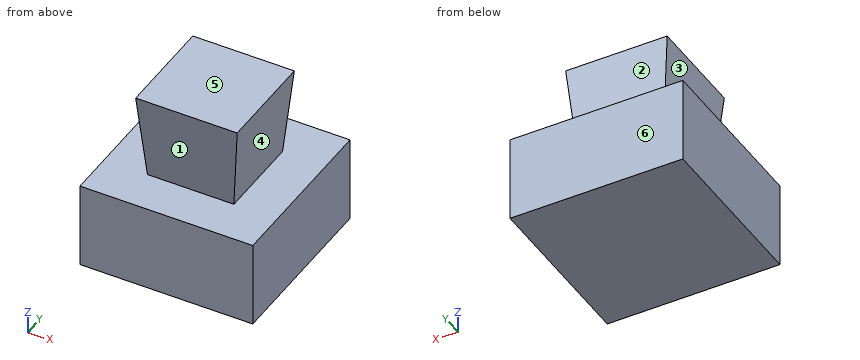
from build123d import *

# Parameters (mm, degrees)
SKETCH_1_W         = 20
SKETCH_1_H         = 20
BASEBOX_DEPTH      = 10
SKETCH_2_W         = 10
SKETCH_2_H         = 10
DRAFTOUTWARD_DEPTH = 10
DRAFTOUTWARD_DRAFT = -5


with BuildPart() as part:
    # 草图1 → BaseBox (new body)
    with BuildSketch(Plane.XY):
        with Locations((10, 10)):
            Rectangle(SKETCH_1_W, SKETCH_1_H)
    extrude(amount=BASEBOX_DEPTH)


with BuildPart() as draftoutward_tool:
    # 草图2 → DraftOutward (with draft: the straight prism first)
    with BuildSketch(Plane.XY.offset(10)):
        with Locations((10, 10)):
            Rectangle(SKETCH_2_W, SKETCH_2_H)
    extrude(amount=DRAFTOUTWARD_DEPTH)
    # DraftOutward: the draft: its side faces are tilted about the plane it starts from
    draftoutward_sides = [draftoutward_tool.faces().sort_by_distance(p)[0] for p in [
        (10, 5, 15),
        (15, 10, 15),
        (10, 15, 15),
        (5, 10, 15),
    ]]
    draft(draftoutward_sides, Plane.XY.offset(10), DRAFTOUTWARD_DRAFT)


with BuildPart() as part_1:
    add(part.part)

    # DraftOutward: add draftoutward_tool
    add(draftoutward_tool.part)


solid = part_1.part
Input: part model. Units: mm. Frame: model coordinates. Face numbers are marked on the shaded views. A direction names the side the tool comes from. Coordinates: 2 decimals unless noted, no trailing zeros. Loops run counter-clockwise (first coordinate to the right, second up) from the corner with the lowest first, then second, coordinate; pieces in that order, holes last. Notation, with made-up numbers: (0, -4.5) -> (45, -4.5) arc R30 cw to (45, 28.5) -> close; hole circle Ø6 at (14.25, 47.25). An arc over 180 degrees is marked (long way). Write each question's results on one line, items separated by ' | '. Start each with the question number.
Q1. Pin query (flat end, axial travel): pin 1 (1 mm diameter, centred on y = 9.5, z = 15, fed in from +X); pin 2 (1.5 mm diameter, centred on x = 3, y = 10, fed in from +Z); pin 3 (10 mm diameter, centred on y = 12, z = 17, fed in from +X). Return the tip coordinate at first contact, or that it passes through.
Q2. Ray query, line 1 (Z direction, x = 16.75, y = 19.25); line 2 (Y direction, x = 15.5, z = 16.25); line 3 (Y direction, x = 6.25, z = 18.75). Return the intervals inside material, ascending. Write a range as from..to.
Q3. Reachability of the marked faces 1, 2 and 3 from +Z, -Z, +X, -X, +Y, -Y: full face, straight path, thin tool, end or side. Return the list, or none.
Q4. Section A-A, the plane x = 4.5. Return the cut outline in (y, z).
Q5. Section B-B, the plane x = 9.75. Return the cut outline in (y, z), plus the area to 3 significant figures.
Q6. Pull-direction query (Z, two-part tool) for the marked faces 4, 5 and 6; classes: released by +Z, released by -Z, zero draft, split by the parting line, or undercut.
Q7. Section D-D, the plane z = 10.5. Return the cut outline in (x, y), plus the area to 3 significant figures.
Found:
1) pin 1: x = 15.48 | pin 2: z = 10 | pin 3: x = 15.87
2) line 1: 0..10 | line 2: 4.45..15.55 | line 3: 4.23..15.77
3) face 1: +X, -X, -Y | face 2: +X, -X, +Y | face 3: -X, +Y, -Y
4) outline: (0, 0) -> (20, 0) -> (20, 10) -> (0, 10) -> close; (4.13, 20) -> (4.5, 15.72) -> (15.5, 15.72) -> (15.87, 20) -> close
5) outline: (0, 0) -> (20, 0) -> (20, 10) -> (15, 10) -> (15.87, 20) -> (4.13, 20) -> (5, 10) -> (0, 10) -> close | area: 309 mm2
6) face 4: undercut | face 5: released by +Z | face 6: zero draft
7) outline: (4.96, 4.96) -> (15.04, 4.96) -> (15.04, 15.04) -> (4.96, 15.04) -> close | area: 102 mm2
